Check sheet for the modelled part. Datum: model origin and axes. Units: mm. A direction names the side the tool comes from. Coordinates: 2 decimals unless noted, no trailing zeros. Write each loop counter-clockwise with the first axis right and the second up, starting at its lowest first coordinate (ties: lowest second). Pieces come first, ordered by that corner, then holes. Notation, with made-up numbers: (13, 75.5) -> (64, 75.5) arc R29 cw to (64, 109.5) -> close; hole circle Ø8 at (-4.5, 83.5). An arc over 180 degrees is marked (long way). Put each result on its own line as item: value.
```python
from build123d import *

# Parameters (mm, degrees)
SKETCH_W        = 8
SKETCH_H        = 58
PAD_DEPTH       = 3
SKETCH001_W     = 8
SKETCH001_H     = 26
PAD001_DEPTH    = 6
SKETCH002_R     = 2
POCKET_DEPTH    = 5
SKETCH003_R     = 3.1
POCKET001_DEPTH = 1


with BuildPart() as part:
    # Sketch → Pad (new body)
    with BuildSketch(Plane.XY):
        with Locations((4, 29)):
            Rectangle(SKETCH_W, SKETCH_H)
    extrude(amount=PAD_DEPTH)

    # Sketch001 (on Face6 of Pad) → Pad001 (join)
    with BuildSketch(Plane.XY.offset(3)):
        with Locations((4, 29)):
            Rectangle(SKETCH001_W, SKETCH001_H)
    extrude(amount=PAD001_DEPTH)

    # Sketch002 (on Face4 of Pad001) → Pocket (cut)
    with BuildSketch(Plane(origin=(0, 0, 0), x_dir=(1, 0, 0), z_dir=(0, 0, -1))):
        with Locations((4, -4)):
            Circle(SKETCH002_R)
        with Locations((4, -54)):
            Circle(SKETCH002_R)
    extrude(amount=-POCKET_DEPTH, mode=Mode.SUBTRACT)

    # Sketch003 (on Face5 of Pocket) → Pocket001 (cut)
    with BuildSketch(Plane.XY.offset(3)):
        with Locations((4, 4)):
            Circle(SKETCH003_R)
        with Locations((4, 54)):
            Circle(SKETCH003_R)
    extrude(amount=-POCKET001_DEPTH, mode=Mode.SUBTRACT)


solid = part.part
```
Q1. Cross-section at A-A (x = 4). Record the cut outline in (y, z).
Recorded:
outline: (0, 0) -> (2, 0) -> (2, 2) -> (0.9, 2) -> (0.9, 3) -> (0, 3) -> close; (6, 0) -> (52, 0) -> (52, 2) -> (50.9, 2) -> (50.9, 3) -> (42, 3) -> (42, 9) -> (16, 9) -> (16, 3) -> (7.1, 3) -> (7.1, 2) -> (6, 2) -> close; (56, 0) -> (58, 0) -> (58, 3) -> (57.1, 3) -> (57.1, 2) -> (56, 2) -> close
Q2. Tool access check on faces 1 (the flat face through (8, 29, 3)), 2 (the cylindrical face through (3.596, 57.074, 2.507)), 3 (the flat face through (4, 42, 6)), 4 (the flat face through (4, 10, 3)). Record the directions out of +Z, -Z, +X, -X, +Y, -Y that give a thin tool (end or side, any length) a straight path to the whole face; none if there is none.
Recorded:
face 1: +Z, -Z, +X, +Y, -Y
face 2: +Z
face 3: +Z, +X, -X, +Y
face 4: +Z, +X, -X, -Y
Q3. Material ranges on line 1 along Y through (x, z) = (4, 1); line 2 along Y through (x, z) = (4, 2.7); line 3 along X through (y, z) = (4, 0.8), recorded low to high.
Recorded:
line 1: y = 0 to 2, 6 to 52, 56 to 58
line 2: y = 0 to 0.9, 7.1 to 50.9, 57.1 to 58
line 3: x = 0 to 2, 6 to 8
Q4. Cross-section at B-B (y = 4). Record the cut outline in (x, z), plus the area to 3 significant figures.
Recorded:
outline: (0, 0) -> (2, 0) -> (2, 2) -> (0.9, 2) -> (0.9, 3) -> (0, 3) -> close; (6, 0) -> (8, 0) -> (8, 3) -> (7.1, 3) -> (7.1, 2) -> (6, 2) -> close
area: 9.80 mm2
Q5. Mould release check, pull along Y, two halves, no side actions. Record for faces 5 (the flat face through (4, 58, 1)), 6 (the flat face through (4, 48, 3)), 7 (the flat face through (4, 16, 6)), 8 (the cylindrical face through (2.526, 52.648, 0.986)): released by +Y, released by -Y, zero draft, split by the parting line, or undercut.
Recorded:
face 5: released by +Y
face 6: zero draft
face 7: released by -Y
face 8: undercut
Q6. Cross-section at D-D (z = 4.5). Record the cut outline in (x, y).
Recorded:
outline: (0, 16) -> (8, 16) -> (8, 42) -> (0, 42) -> close
Q7. Cross-section at C-C (z = 1.25). Record the cut outline in (x, y), plus the area to 3 significant figures.
Recorded:
outline: (0, 0) -> (8, 0) -> (8, 58) -> (0, 58) -> close; hole circle Ø4 at (4, 4); hole circle Ø4 at (4, 54)
area: 439 mm2
Q8. Depth check by flat-ended pin: P1, Ø3, axis at x = 5.5, z = 6, coming from the +Y side; P2, Ø4, axis at x = 2.5, y = 48, coming from the +Z side; P3, Ø3.5, axis at x = 4, y = 4, coming from the +Z side; P4, Ø4.5, axis at x = 4, y = 54, coming from the +Z side. Enter the tip coordinate at first touch or a pass-through.
Recorded:
P1: stops at y = 42
P2: stops at z = 3
P3: passes through
P4: stops at z = 2
